Input: dimensioned drawing with shaded views. Units: mm. Origin: part minimum x, y, z. A direction names the side the tool comes from. Coordinates: 2 decimals unless noted, no trailing zeros. Order: outer loops, then holes, each group sorted by start corner. A loop starts at its lowest first (then second) coordinate and runs counter-clockwise, first axis right, second up. Notation, with made-up numbers: (-29, 63) -> (-16, 63) arc R9 ccw to (-16, 71) -> close; hole circle Ø3 at (-19.5, 7). An arc over 180 degrees is marked (long way). Put each result on its own line as item: value.
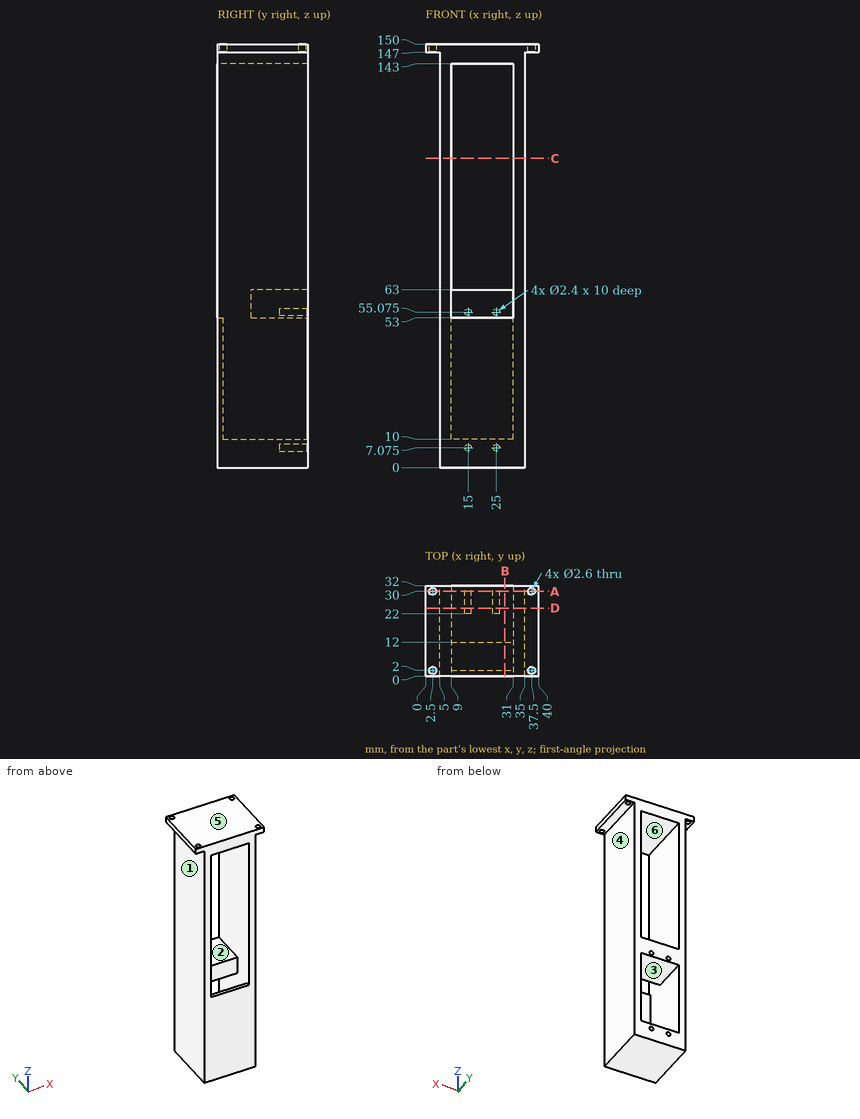
1. Ray query, line 1 along Z through (x, y) = (19, 13); line 2 along Z through (x, y) = (30, 5.5); line 3 along Y through (x, z) = (2.5, 147.95). Return the intervals inside material, ascending.
Numbers:
line 1: z = 0 to 10, 53 to 63, 143 to 150
line 2: z = 0 to 10, 143 to 150
line 3: y = 0 to 0.7, 3.3 to 28.7, 31.3 to 32
2. Set-up query: the marked faces 1, 2 and 3. Return all of +Z, -Z, +X, -X, +Y, -Y with unobstructed straight access to the full face (end or side cutting, diameter ignored); none if empty.
Numbers:
face 1: -Z, -X, +Y, -Y
face 2: +Y, -Y
face 3: +Y
3. First-contact query: pin 1 (9.5 mm diameter, centred on y = 15.5, z = 68, fed in from +X); pin 2 (4 mm diameter, centred on x = 2.5, y = 2, fed in from -Z); pin 3 (1.6 mm diameter, centred on x = 2.5, y = 30, fed in from +Z); pin 4 (1.4 mm diameter, centred on x = 25, z = 7.08, fed in from +Y). Flat tips, straight axial feed; report the tip coordinate or a pass-through.
Numbers:
pin 1: stops at x = 35
pin 2: stops at z = 147
pin 3: passes through
pin 4: stops at y = 22
4. Cut plane A-A on y = 30. Count the separate pieces of the cut face and the enclosed holes in it, plus the area to 3 significant figures.
Numbers:
separate pieces: 3
enclosed holes: 6
area: 1,790 mm2
5. Cut plane B-B on x = 28. Output: boundary loops of the cut face in (y, z), plus the area to 3 significant figures.
Numbers:
outline: (0, 0) -> (32, 0) -> (32, 10) -> (2, 10) -> (2, 53) -> (0, 53) -> close; (0, 143) -> (32, 143) -> (32, 150) -> (0, 150) -> close; (12, 53) -> (32, 53) -> (32, 63) -> (12, 63) -> close
area: 830 mm2
6. Pull-direction query (X, two-part tool) for the marked faces 4, 5 and 6; classes: pulls with the +X half, pulls with the -X half, needs draft (parallel to the pull), parting line crosses it, or undercut.
Numbers:
face 4: pulls with the +X half
face 5: needs draft
face 6: undercut
7. Cut plane D-D on y = 24. Output: boundary loops of the cut face in (x, z) (1 decimal), plus the area to 3 significant figures.
Numbers:
outline: (0, 147) -> (5, 147) -> (5, 0) -> (35, 0) -> (35, 147) -> (40, 147) -> (40, 150) -> (0, 150) -> close; hole (9, 10) -> (31, 10) -> (31, 53) -> (9, 53) -> close; hole (9, 63) -> (31, 63) -> (31, 143) -> (9, 143) -> close; hole circle Ø2.4 at (15, 7.1); hole circle Ø2.4 at (15, 55.1); hole circle Ø2.4 at (25, 7.1); hole circle Ø2.4 at (25, 55.1)
area: 1,810 mm2
8. Cut plane C-C on z = 109.5. Output: boundary loops of the cut face in (x, y).
Numbers:
outline: (5, 0) -> (9, 0) -> (9, 32) -> (5, 32) -> close; (31, 0) -> (35, 0) -> (35, 32) -> (31, 32) -> close
